Geometry: see drawing. Coordinates: mm, zero at the bounding-box minimum. A direction names the side the tool comes from. Coordinates: 2 decimals unless noted, no trailing zeros. Loops run counter-clockwise (first coordinate to the right, second up) from the corner with the lowest first, then second, coordinate; pieces in that order, holes last. Notation, with made-up numbers: (-40, 4.25) -> (-23, 4.25) arc R12 ccw to (-23, 17.25) -> close; hole circle Ø2 at (24, 31). An arc over 180 degrees is marked (long way). Answer as a JSON object with one key per item and string values.
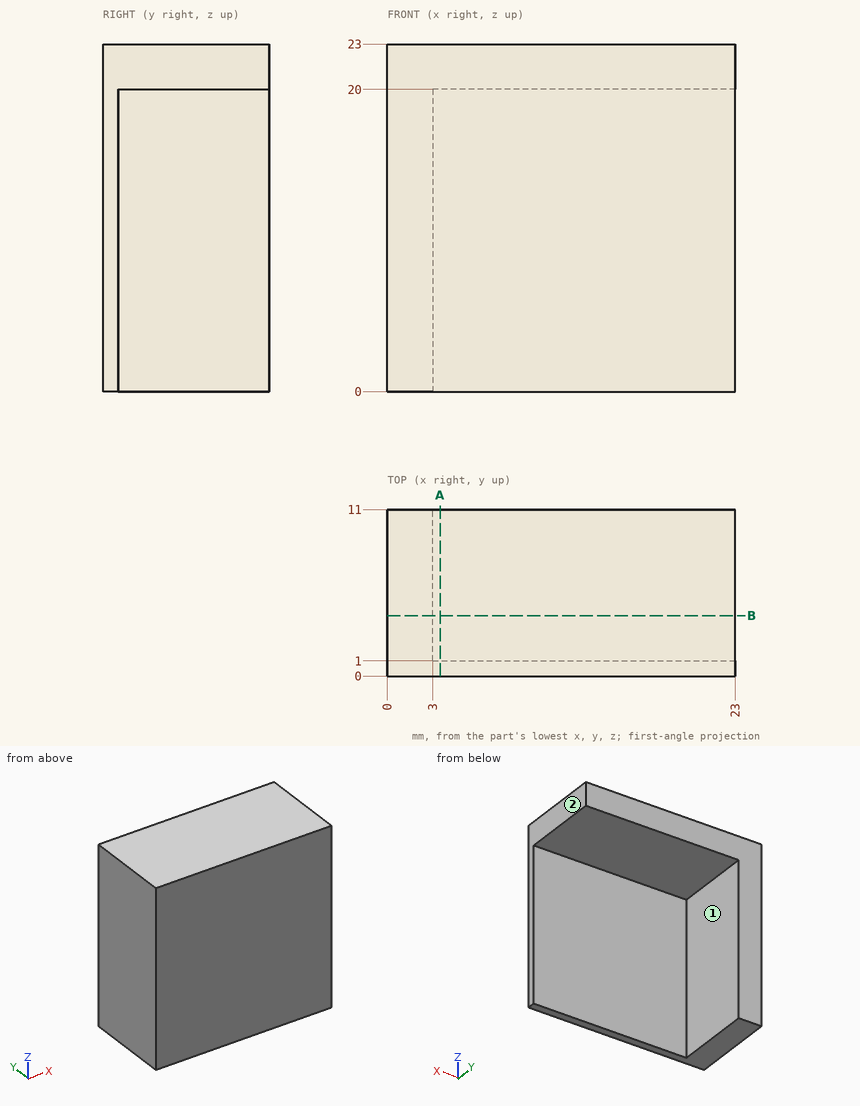
1. Section query A-A (x = 3.5). Return loops of the section in (y, z).
Reply:
{"outline": "(0, 0) -> (1, 0) -> (1, 20) -> (11, 20) -> (11, 23) -> (0, 23) -> close"}
2. Line query: line 1 along Y through (x, z) = (19.75, 4); line 2 along X through (y, z) = (7, 3.75); line 3 along Z through (x, y) = (13.25, 2.25). Output: solid intervals per line, ascending.
Reply:
{"line 1": "y = 0 to 1", "line 2": "x = 0 to 3", "line 3": "z = 20 to 23"}
3. Section query B-B (y = 4). Return loops of the section in (x, z).
Reply:
{"outline": "(0, 0) -> (3, 0) -> (3, 20) -> (23, 20) -> (23, 23) -> (0, 23) -> close"}
4. Pin query (flat end, axial travel): P1, Ø3, axis at x = 14.5, y = 6.5, coming from the -Z side; P2, Ø6, axis at x = 13, z = 13.5, coming from the +Y side. Return the tip coordinate at first contact, or that it passes through.
Reply:
{"P1": "stops at z = 20", "P2": "stops at y = 1"}
5. Access query for the marked faces 1 and 2. Directions: +Z, -Z, +X, -X, +Y, -Y. A direction counts if a zero-diameter tool reaches every point of the face in a straight line with its end or side. Return the directions, or none.
Reply:
{"face 1": "-Z, +X, +Y", "face 2": "+Z, -Z, +X, +Y, -Y"}
